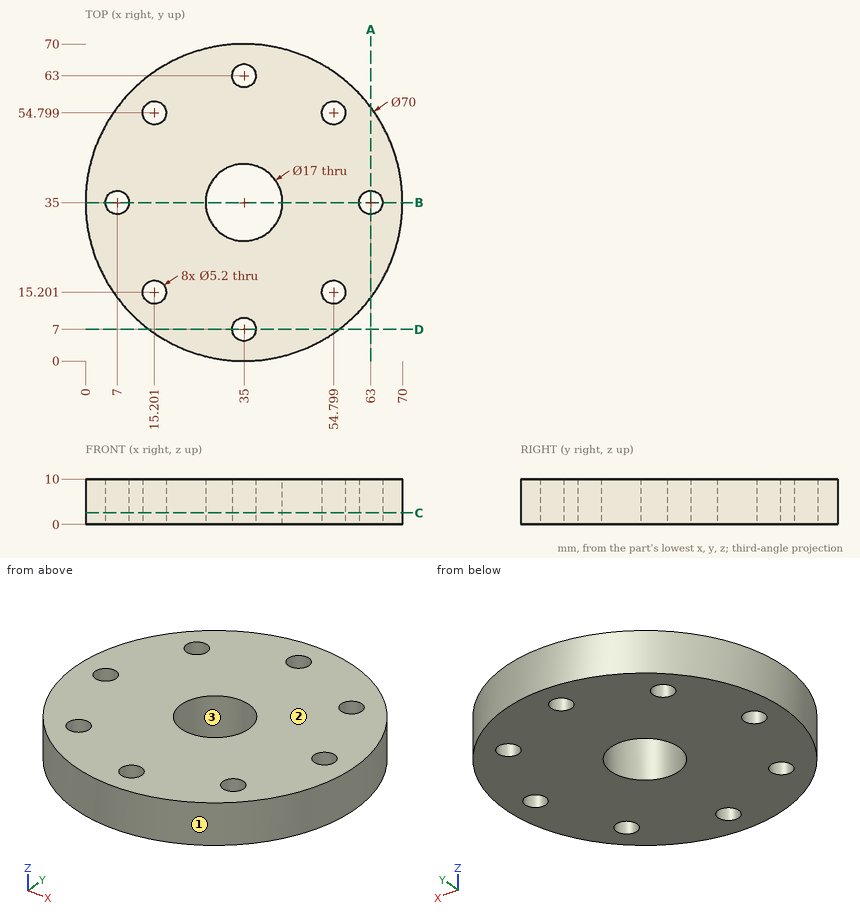
Verification items for this drawing (mm, ordinates from the low corner). Coordinates: 2 decimals unless noted, no trailing zeros. Loops run counter-clockwise (first coordinate to the right, second up) from the corner with the lowest first, then second, coordinate; pieces in that order, holes last. Notation, with made-up numbers: (83.25, 84) -> (119.25, 84) arc R24 ccw to (119.25, 103) -> close; hole circle Ø8 at (-34, -5). An arc over 180 degrees is marked (long way). Answer in a Markdown table with one row per item. Add a question column.
1. Section check C-C, the plane z = 2.5. Give the number of separate pieces and of enclosed holes in the cut face, then the cut area to 3 significant figures.
2. Section check B-B, the plane y = 35. Enter the section's corners in (x, z).
3. Depth check by flat-ended pin: P1, Ø8.5, axis at x = 63, y = 35, coming from the +Z side; P2, Ø2, axis at y = 23, z = 2.5, coming from the +X side; P3, Ø4, axis at x = 42.5, z = 4.5, coming from the -Y side; P4, Ø3, axis at x = 48.5, z = 2, coming from the +Y side. Enter the tip coordinate at first touch or a pass-through.
4. Material ranges on probe 1 along Y at (x, z) = (39, 1.25); probe 2 along Y at (x, z) = (61.5, 6.5); probe 3 along X at (y, z) = (7, 4.5), recorded low to high. Write a range as [from, to].
5. Section check A-A, the plane x = 63. Enter the section's corners in (y, z).
6. Draft check along Y on the marked faces 1, 2 and 3. Enter one of: +Y half, -Y half, draft (parallel to the pull), parting line (faces both ways), or undercut.
Derived:
| question | item | result |
|---|---|---|
| 1 | separate pieces | 1 |
| 1 | enclosed holes | 9 |
| 1 | area | 3,450 mm² |
| 2 | outline | (0, 0) -> (4.4, 0) -> (4.4, 10) -> (0, 10) -> close; (9.6, 0) -> (26.5, 0) -> (26.5, 10) -> (9.6, 10) -> close; (43.5, 0) -> (60.4, 0) -> (60.4, 10) -> (43.5, 10) -> close; (65.6, 0) -> (70, 0) -> (70, 10) -> (65.6, 10) -> close |
| 3 | P1 | stops at z = 10 |
| 3 | P2 | stops at x = 68.23 |
| 3 | P3 | stops at y = 0.43 |
| 3 | P4 | stops at y = 67.88 |
| 4 | probe 1 | y = [0.23, 27.5], [42.5, 69.77] |
| 4 | probe 2 | y = [12.14, 32.88], [37.12, 57.86] |
| 4 | probe 3 | x = [14, 32.4], [37.6, 56] |
| 5 | outline | (14, 0) -> (32.4, 0) -> (32.4, 10) -> (14, 10) -> close; (37.6, 0) -> (56, 0) -> (56, 10) -> (37.6, 10) -> close |
| 6 | face 1 | parting line |
| 6 | face 2 | draft |
| 6 | face 3 | undercut |
